Part print with two shaded views. Sizes in mm from the minimum x, y, z corner. A direction names the side the tool comes from. Round coordinates to 2 decimals unless told otherwise and drop trailing zeros. Write each loop counter-clockwise with the first axis right and the second up, starting at its lowest first coordinate (ties: lowest second). Pieces come first, ordered by that corner, then holes. Notation, with made-up numbers: (67.5, 30) -> (99.5, 30) arc R24 ccw to (99.5, 62) -> close; hole circle Ø3 at (66.5, 80.5). An arc over 180 degrees is marked (long way). Put each result on its own line as item: value. Start each with the question number.
1. Saw through at C-C on y = 15.25. List the corners of the cut face in (x, z), and give its area (3 significant figures).
2. Flat gauge pins, fed straight in: P1, Ø12, axis at y = 18.5, z = 19.5, coming from the +X side; P2, Ø5, axis at x = 2.5, z = 7, coming from the -Y side; P3, Ø3, axis at y = 9.5, z = 17.5, coming from the -X side; P4, Ø4, axis at x = 11.5, z = 12, coming from the +Y side. Where does each tip first touch, or does it go through?
3. Saw through at B-B on z = 28. List the corners of the cut face in (x, y) (1 decimal).
4. 3-axis set-ups, long thin cutter, end or side, ignore diameter. For the marked faces 1 and 2: which of +Z, -Z, +X, -X, +Y, -Y reach the whole face in a straight line?
5. Pull direction Z, two halves, no side cores. Call the marked faces 3, 4 and 5: pulls with the +Z half, pulls with the -Z half, needs draft (parallel to the pull), parting line crosses it, or undercut.
6. Drill centre lines: line 1 (Z direction, x = 15.5, y = 5.75); line 2 (X direction, y = 11, z = 14.5); line 3 (Z direction, x = 6.5, y = 9.5). Where is each one in solid material? Low to high. Write a range as from..to.
7. Saw through at D-D on x = 8. List the corners of the cut face in (y, z), and give its area (3 significant figures).
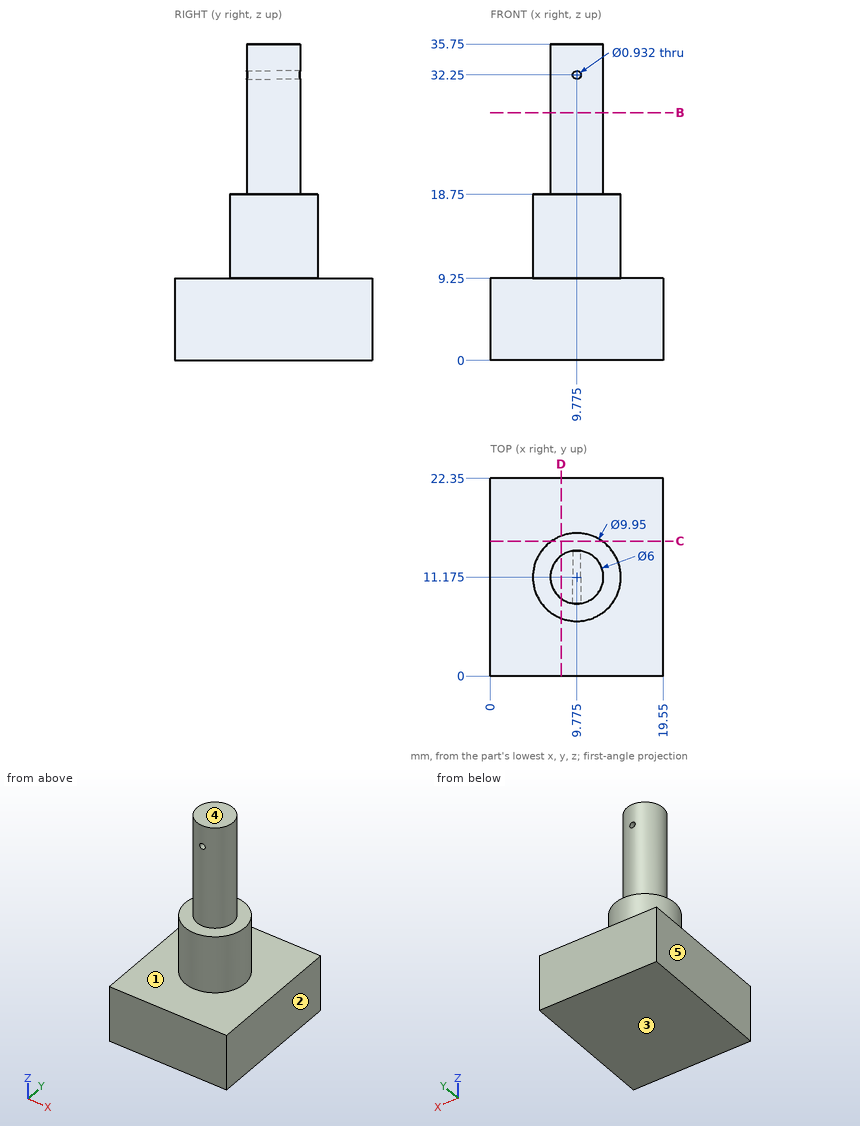
Return value:
1. outline: (0, 0) -> (19.55, 0) -> (19.55, 9.25) -> (12.63, 9.25) -> (12.63, 18.75) -> (6.92, 18.75) -> (6.92, 9.25) -> (0, 9.25) -> close
1. area: 235 mm^2
2. P1: stops at x = 14.56
2. P2: stops at y = 0
2. P3: stops at x = 4.8
2. P4: stops at y = 16.15
3. outline: circle Ø6 at (9.8, 11.2)
4. face 1: +Z
4. face 2: +Z, -Z, +X, +Y, -Y
5. face 3: pulls with the -Z half
5. face 4: pulls with the +Z half
5. face 5: needs draft
6. line 1: z = 0..9.25
6. line 2: x = 4.8..14.75
6. line 3: z = 0..18.75
7. outline: (0, 0) -> (22.35, 0) -> (22.35, 9.25) -> (15.82, 9.25) -> (15.82, 18.75) -> (13.59, 18.75) -> (13.59, 35.75) -> (8.76, 35.75) -> (8.76, 18.75) -> (6.53, 18.75) -> (6.53, 9.25) -> (0, 9.25) -> close
7. area: 377 mm^2
